```python
from build123d import *

# Parameters (mm, degrees)
F0_R     = 12.7
F1_DEPTH = 6.35
F2_W     = 38.1
F2_H     = 6.35
F3_DEPTH = 50.8
F4_R     = 6.35
F5_DEPTH = 25.4


with BuildPart() as f1:
    # F0 (on Front) → F1 (new body)
    with BuildSketch(Plane.XZ):
        Polygon((44.45, 57.15), (-107.95, 57.15), (-107.95, -59.163763), (-31.618457, -59.163763), (-31.618457, -72.087309), (-107.95, -72.087309), (-107.95, -146.05), (-69.85, -146.05), (-69.85, -126.62439), (6.35, -126.62439), (6.35, -146.05), (44.45, -146.05), align=None)
        Circle(F0_R, mode=Mode.SUBTRACT)
    extrude(amount=F1_DEPTH)

    # F2 (on face) → F3 (join)
    with BuildSketch(Plane(origin=(0, 0, 0), x_dir=(-1, 0, 0), z_dir=(0, 1, 0))):
        with Locations((-25.4, -142.875)):
            Rectangle(F2_W, F2_H)
        with Locations((88.9, -142.875)):
            Rectangle(F2_W, F2_H)
    extrude(amount=F3_DEPTH)

    # F4 (on face) → F5 (cut)
    with BuildSketch(Plane.XY.offset(-139.7)):
        with Locations((26.022155, 25.4)):
            Circle(F4_R)
        with Locations((-90.712979, 26.081869)):
            Circle(F4_R)
    extrude(amount=-F5_DEPTH, mode=Mode.SUBTRACT)


solid = f1.part
```
Geometry check sheet. Reference: the model listing, model coordinates, mm. A direction names the side the tool comes from. Give positions to 0.01 mm unless a question says otherwise; leave off trailing zeros. Write each loop counter-clockwise with the first axis right and the second up, starting at its lowest first coordinate (ties: lowest second). Pieces come first, ordered by that corner, then holes.
1) Section check B-B, the plane x = 0. Record the boundary of the cut face in (y, z).
2) Material ranges on L1, parallel to Z at x = 0, y = -1.5; L2, parallel to Z at x = -76, y = -3.5; L3, parallel to X at y = 25, z = -144, recorded low to high.
3) Release check for a two-part mould opening along X. For faces 1 (the flat face through (-107.95, -1, -123)), 2 (the flat face through (-32, -3, -126.624)), 3 (the flat face through (-84.9, 22.6, -146.05)) record: pulls with the +X half, pulls with the -X half, needs draft (parallel to the pull), parting line crosses it, or undercut.
4) Section check A-A, the plane y = 8.5. Record the boundary of the cut face in (x, z).
5) Section check C-C, the plane z = -15. Record the boundary of the cut face in (x, y), and give its area (3 significant figures).
6) Gauge pin test, flat ends, axial feed: pin 1 (6 mm diameter, centred on x = -51.5, y = 3.5, fed in from +Z); pin 2 (1.9 mm diameter, centred on y = -2.5, z = -65.5, fed in from -X); pin 3 (19 mm diameter, centred on x = 16.5, y = 31.5, fed in from +Z); pin 4 (3 mm diameter, centred on x = -30, y = -2, fed in from -Z). Record the tip position at first contact, or that the pin passes through.
7) Section check D-D, the plane x = 30. Record the boundary of the cut face in (y, z), and give its area (3 significant figures).
8) Access from +Z, -Z, +X, -X, +Y, -Y to the whole of each face (thin tool, end or side, straight path). Record for faces 4 (the flat face through (-70, -3, -59.164)), 5 (the flat face through (-84, 25, -139.7)), 6 (the flat face through (-69.85, 16, -141)), 7 (the cylindrical face through (31.9, 23, -142.8)).
Computed:
1. outline: (-6.35, -126.62) - (0, -126.62) - (0, -12.7) - (-6.35, -12.7) - close; (-6.35, 12.7) - (0, 12.7) - (0, 57.15) - (-6.35, 57.15) - close
2. L1: z = -126.62 to -12.7, 12.7 to 57.15
2. L2: z = -146.05 to -72.09, -59.16 to 57.15
2. L3: x = -107.95 to -96.97, -84.46 to -69.85, 6.35 to 19.68, 32.36 to 44.45
3. face 1: pulls with the -X half
3. face 2: undercut
3. face 3: needs draft
4. outline: (-107.95, -146.05) - (-69.85, -146.05) - (-69.85, -139.7) - (-107.95, -139.7) - close; (6.35, -146.05) - (44.45, -146.05) - (44.45, -139.7) - (6.35, -139.7) - close
5. outline: (-107.95, -6.35) - (44.45, -6.35) - (44.45, 0) - (-107.95, 0) - close
5. area: 968 mm2
6. pin 1: passes through
6. pin 2: stops at x = -31.62
6. pin 3: stops at z = -139.7
6. pin 4: stops at z = -126.62
7. outline: (-6.35, -146.05) - (20.45, -146.05) - (20.45, -139.7) - (0, -139.7) - (0, 57.15) - (-6.35, 57.15) - close; (30.35, -146.05) - (50.8, -146.05) - (50.8, -139.7) - (30.35, -139.7) - close
7. area: 1,550 mm2
8. face 4: -X, +Y, -Y
8. face 5: +Z, +X, -X, +Y
8. face 6: -Z, +Y, -Y
8. face 7: +Z, -Z
